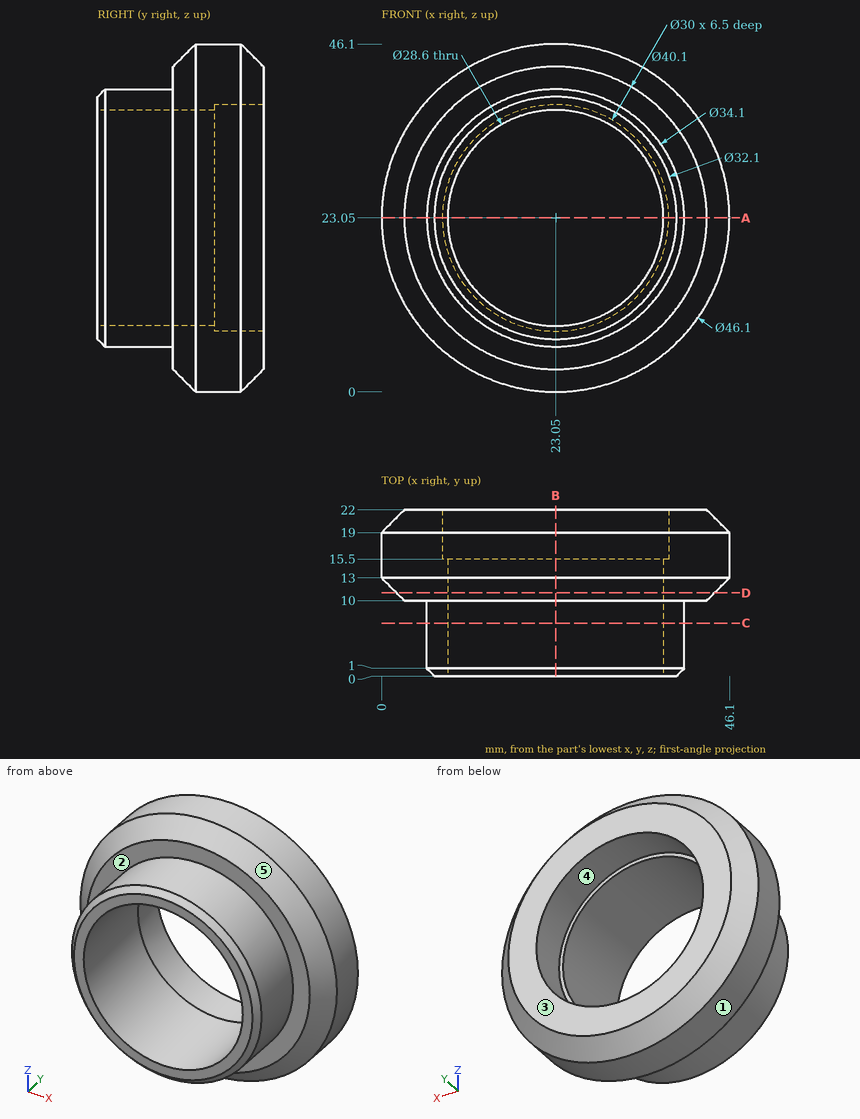
Check sheet for the drawn part. Datum: minimum x, y, z corner. Units: mm. A direction names the side the tool comes from. Round coordinates to 2 decimals unless told otherwise and drop trailing zeros. Order: outer loops, then holes, each group sorted by start corner. A loop starts at its lowest first (then second) coordinate and runs counter-clockwise, first axis right, second up. Notation, with made-up numbers: (50.5, 66.25) - (64.5, 66.25) arc R6 cw to (64.5, 73.25) - close; hole circle Ø11 at (33.5, -7). An arc over 180 degrees is marked (long way). Use a Markdown table: item, result. Add a question column.
(1) Sectioned sample at B-B, the plane x = 23.05. Enter the section's corners in (y, z).
(2) Tool access check on the marked faces 1 and 2. Record the directions out of +Z, -Z, +X, -X, +Y, -Y that give a thin tool (end or side, any length) a straight path to the whole face; none if there is none.
(3) Sectioned sample at D-D, the plane y = 11. Enter the section's corners in (x, z), and give its area (3 significant figures).
(4) Sectioned sample at C-C, the plane y = 7. Enter the section's corners in (x, z).
(5) Depth check by flat-ended pin: pin 1 (8 mm diameter, centred on x = 14, y = 8.5, fed in from -Z); pin 2 (5 mm diameter, centred on x = 21, y = 20, fed in from -Z); pin 3 (1.5 mm diameter, centred on y = 15, z = 39, fed in from -X). Enter the tip coordinate at first touch or a pass-through.
(6) Release check for a two-part mould opening along X. For the marked faces 3, 4 and 5 record: pulls with the +X half, pulls with the -X half, needs draft (parallel to the pull), parting line crosses it, or undercut.
(7) Sectioned sample at A-A, the plane z = 23.05. Enter the section's corners in (x, y).
(8) Material ranges on line 1 along Z through (x, y) = (23.05, 6.5); line 2 along Z through (x, y) = (23.05, 20.5); line 3 along X through (y, z) = (10.25, 31), recorded low to high. Write a range as [from, to].
Answers below:
| question | item | result |
|---|---|---|
| 1 | outline | (0, 7) - (1, 6) - (10, 6) - (10, 3) - (13, 0) - (19, 0) - (22, 3) - (22, 8.05) - (15.5, 8.05) - (15.5, 8.75) - (0, 8.75) - close; (0, 37.35) - (15.5, 37.35) - (15.5, 38.05) - (22, 38.05) - (22, 43.1) - (19, 46.1) - (13, 46.1) - (10, 43.1) - (10, 40.1) - (1, 40.1) - (0, 39.1) - close |
| 2 | face 1 | +Y, -Y |
| 2 | face 2 | -Y |
| 3 | outline | circle Ø42.1 at (23.05, 23.05); hole circle Ø28.6 at (23.05, 23.05) |
| 3 | area | 750 mm² |
| 4 | outline | circle Ø34.1 at (23.05, 23.05); hole circle Ø28.6 at (23.05, 23.05) |
| 5 | pin 1 | z = 2.1 |
| 5 | pin 2 | z = 0 |
| 5 | pin 3 | x = 5.72 |
| 6 | face 3 | needs draft |
| 6 | face 4 | undercut |
| 6 | face 5 | parting line crosses it |
| 7 | outline | (0, 13) - (3, 10) - (6, 10) - (6, 1) - (7, 0) - (8.75, 0) - (8.75, 15.5) - (8.05, 15.5) - (8.05, 22) - (3, 22) - (0, 19) - close; (37.35, 0) - (39.1, 0) - (40.1, 1) - (40.1, 10) - (43.1, 10) - (46.1, 13) - (46.1, 19) - (43.1, 22) - (38.05, 22) - (38.05, 15.5) - (37.35, 15.5) - close |
| 8 | line 1 | [6, 8.75], [37.35, 40.1] |
| 8 | line 2 | [1.5, 8.05], [38.05, 44.6] |
| 8 | line 3 | [4.37, 11.16], [34.94, 41.73] |
